The model under review builds one solid part; all positions refer to its coordinate system, in mm. Face numbers are marked on the shaded views. A direction names the side the tool comes from. Coordinates: 2 decimals unless noted, no trailing zeros. Write each loop counter-clockwise with the first axis right and the second up, starting at its lowest first coordinate (ties: lowest second). Pieces come first, ordered by that corner, then holes. Notation, with made-up numbers: (77, 39) -> (128, 39) arc R25 cw to (128, 55) -> close; hole circle Ø8 at (-28.75, 76.5). An arc over 180 degrees is marked (long way). Put each result on its own line as item: value. Start each with the question number.
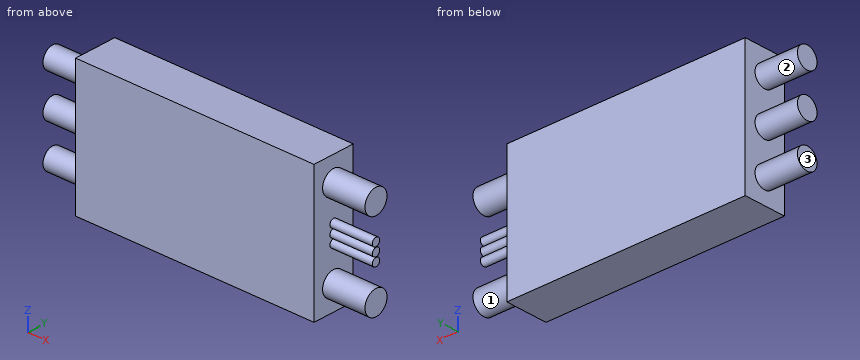
from build123d import *

# Parameters (mm, degrees)
SKETCH1_W           = 45
SKETCH1_H           = 25
BOSS_EXTRUDE1_DEPTH = 8
SKETCH2_R           = 2
BOSS_EXTRUDE2_DEPTH = 8
SKETCH3_R           = 2.25
SKETCH3_R_2         = 0.75
BOSS_EXTRUDE5_DEPTH = 8


with BuildPart() as part:
    # Sketch1 → Boss-Extrude1 (new body)
    with BuildSketch(Plane(origin=(0, 0, 0), x_dir=(1, 0, 0), z_dir=(0, 1, 0))):
        with Locations((22.5, 12.5)):
            Rectangle(SKETCH1_W, SKETCH1_H)
    extrude(amount=BOSS_EXTRUDE1_DEPTH)

    # Sketch2 → Boss-Extrude2 (add)
    with BuildSketch(Plane.ZY):
        with Locations((-12.5, 4)):
            Circle(SKETCH2_R)
        with Locations((-20.5, 4)):
            Circle(SKETCH2_R)
        with Locations((-4.5, 4)):
            Circle(SKETCH2_R)
    extrude(amount=BOSS_EXTRUDE2_DEPTH)

    # Sketch3 → Boss-Extrude5 (add)
    with BuildSketch(Plane(origin=(45, 0, 0), x_dir=(0, 0, -1), z_dir=(1, 0, 0))):
        with Locations((4.5, 4)):
            Circle(SKETCH3_R)
        with Locations((20.5, 4)):
            Circle(SKETCH3_R)
        with Locations((10.9, 4)):
            Circle(SKETCH3_R_2)
        with Locations((12.5, 4)):
            Circle(SKETCH3_R_2)
        with Locations((14.1, 4)):
            Circle(SKETCH3_R_2)
    extrude(amount=BOSS_EXTRUDE5_DEPTH)


solid = part.part
1. Tool access review of the marked faces 1, 2 and 3: name each direction out of +Z, -Z, +X, -X, +Y, -Y from which nothing blocks a thin tool from reaching the whole face with its end or side.
2. Insertion check: P1, Ø3, axis at x = -0.5, z = -17, coming from the +Y side; P2, Ø1.5, axis at y = 7, z = -18.5, coming from the +X side. Each pin has a flat end and moves straight along its axis. Give the tip position at first contact, or say it passes through.
3. Consider section A-A on z = -12.5. State the section outline as (x, y) points, then the cut area to 3 significant figures.
4. Wall thickness on line 1 (X direction, y = 6, z = -17.25); line 2 (Z direction, x = 46, y = 6); line 3 (X direction, y = 2, z = -3.75): over which ranges is each line inside the solid? List them lowest first. Write a range as from..to.
5. Consider section C-C on y = 7. State the section outline as (x, z) points.
6. Consider section D-D on z = -4.5. State the section outline as (x, y) points.
7. Consider section B-B on x = 48.5. State the section outline as (y, z) points.
Output values:
1. face 1: +X
1. face 2: -X
1. face 3: +Z, -Z, -X, +Y, -Y
2. P1: stops at y = 8
2. P2: stops at x = 45
3. outline: (-8, 2) -> (0, 2) -> (0, 0) -> (45, 0) -> (45, 3.25) -> (53, 3.25) -> (53, 4.75) -> (45, 4.75) -> (45, 8) -> (0, 8) -> (0, 6) -> (-8, 6) -> close
3. area: 404 mm^2
4. line 1: x = 0..45
4. line 2: z = -21.53..-19.47, -5.53..-3.47
4. line 3: x = 0..53
5. outline: (0, -25) -> (45, -25) -> (45, 0) -> (0, 0) -> close
6. outline: (-8, 2) -> (0, 2) -> (0, 0) -> (45, 0) -> (45, 1.75) -> (53, 1.75) -> (53, 6.25) -> (45, 6.25) -> (45, 8) -> (0, 8) -> (0, 6) -> (-8, 6) -> close
7. outline: circle Ø4.5 at (4, -20.5); circle Ø4.5 at (4, -4.5); circle Ø1.5 at (4, -14.1); circle Ø1.5 at (4, -12.5); circle Ø1.5 at (4, -10.9)
